Autodesk Inventor part; units mm, degrees
ref_plane "YZ Plane" through (0, 0, 0) normal (1, 0, 0) x (0, 1, 0)
ref_plane "XZ Plane" through (0, 0, 0) normal (0, 1, 0) x (-1, 0, 0)
ref_plane "XY Plane" through (0, 0, 0) normal (0, 0, 1) x (1, 0, 0)
sketch "Sketch1" plane through (0, 0, 0) normal (0, 1, 0) x (-1, 0, 0)
  line L0 (20, 147) -> (20, 150)
  line L1 (20, 150) -> (40, 150)
  line L2 (40, 150) -> (40, 147)
  line L3 (-20, 147) -> (-20, 150)
  line L4 (-20, 150) -> (-40, 150)
  line L5 (-40, 150) -> (-40, 147)
  line L6 (-40, 147) -> (-57, 147)
  line L7 (57, 147) -> (40, 147)
  line L8 (20, 147) -> (-20, 147)
  line L9 (20, -147) -> (20, -150)
  line L10 (20, -150) -> (40, -150)
  line L11 (40, -150) -> (40, -147)
  line L12 (-40, -147) -> (-40, -150)
  line L13 (-40, -150) -> (-20, -150)
  line L14 (-20, -150) -> (-20, -147)
  line L15 (40, -147) -> (57, -147)
  line L16 (-57, -147) -> (-40, -147)
  line L17 (-20, -147) -> (20, -147)
  line L18 (-57, 131.4286) -> (-60, 131.4286)
  line L19 (-60, 131.4286) -> (-60, 108.5714)
  line L20 (-60, 108.5714) -> (-57, 108.5714)
  line L21 (-57, 11.4286) -> (-60, 11.4286)
  line L22 (-60, 11.4286) -> (-60, -11.4286)
  line L23 (-60, -11.4286) -> (-57, -11.4286)
  line L24 (-57, -108.5714) -> (-60, -108.5714)
  line L25 (-60, -108.5714) -> (-60, -131.4286)
  line L26 (-60, -131.4286) -> (-57, -131.4286)
  line L27 (-57, 147) -> (-57, 131.4286)
  line L28 (-57, -131.4286) -> (-57, -147)
  line L29 (57, 131.4286) -> (60, 131.4286)
  line L30 (60, 131.4286) -> (60, 108.5714)
  line L31 (60, 108.5714) -> (57, 108.5714)
  line L32 (57, 11.4286) -> (60, 11.4286)
  line L33 (60, 11.4286) -> (60, -11.4286)
  line L34 (60, -11.4286) -> (57, -11.4286)
  line L35 (57, -108.5714) -> (60, -108.5714)
  line L36 (60, -108.5714) -> (60, -131.4286)
  line L37 (60, -131.4286) -> (57, -131.4286)
  line L38 (57, 131.4286) -> (57, 147)
  line L39 (57, 11.4286) -> (57, 108.5714)
  line L40 (57, -147) -> (57, -131.4286)
  line L41 (57, -108.5714) -> (57, -11.4286)
  line L42 (-57, 57.1429) -> (-60, 57.1429)
  line L43 (-60, 57.1429) -> (-60, 34.2857)
  line L44 (-60, 34.2857) -> (-57, 34.2857)
  line L45 (-57, -34.2857) -> (-60, -34.2857)
  line L46 (-60, -34.2857) -> (-60, -57.1429)
  line L47 (-60, -57.1429) -> (-57, -57.1429)
  line L48 (-57, 108.5714) -> (-57, 57.1429)
  line L49 (-57, 34.2857) -> (-57, 11.4286)
  line L50 (-57, -11.4286) -> (-57, -34.2857)
  line L51 (-57, -57.1429) -> (-57, -108.5714)
  line L52 (-36, 80) -> (-12, 80)
  line L53 (-12, 80) -> (-12, 83)
  line L54 (-12, 83) -> (-36, 83)
  line L55 (-36, 83) -> (-36, 80)
  line L56 (-36, -80) -> (-12, -80)
  line L57 (-12, -80) -> (-12, -83)
  line L58 (-12, -83) -> (-36, -83)
  line L59 (-36, -83) -> (-36, -80)
  line L60 (12, 83) -> (36, 83)
  line L61 (36, 83) -> (36, 80)
  line L62 (36, 80) -> (12, 80)
  line L63 (12, 80) -> (12, 83)
  line L64 (12, -80) -> (36, -80)
  line L65 (36, -80) -> (36, -83)
  line L66 (36, -83) -> (12, -83)
  line L67 (12, -83) -> (12, -80)
  point P0 (0, 0)
  point P1 (-60, 120)
  point P2 (-60, -120)
  dimension "d1" = 294
  dimension "d5" = 20
  dimension "d7" = 20
  dimension "d9" = 3
  dimension "d10" = 147
  dimension "d11" = 3
  dimension "d12" = 57
  dimension "d13" = 3
  dimension "d14" = 17
  dimension "d15" = 3
  dimension "d16" = 17
  dimension "d17" = 22.8571
  dimension "d18" = 11.4286
  dimension "d20" = 120
  dimension "d21" = 17
  dimension "d24" = 114
  dimension "d25" = 22.8571
  dimension "d26" = 24
  dimension "d27" = 3
  dimension "d28" = 3
  dimension "d29" = 22.8571
  dimension "d30" = 24
  dimension "d31" = 24
  dimension "d32" = 22.8571
  dimension "d33" = 120
extrude "Extrusion1" add sketch "Sketch1" along normal blind 3
sketch "Sketch2" plane through (0, 3, 0) normal (0, 1, 0) x (1, 0, 0)
  line L0 (34.2, 76.5) -> (11.4, 76.5)
  line L1 (11.4, 76.5) -> (11.4, 73.5)
  line L2 (11.4, 73.5) -> (34.2, 73.5)
  line L3 (34.2, 73.5) -> (34.2, 76.5)
  line L4 (-11.4, 76.5) -> (-34.2, 76.5)
  line L5 (-34.2, 76.5) -> (-34.2, 73.5)
  line L6 (-34.2, 73.5) -> (-11.4, 73.5)
  line L7 (-11.4, 73.5) -> (-11.4, 76.5)
  line L8 (34.2, 73.5) -> (57, 73.5) construction
  line L9 (11.4, 73.5) -> (-11.4, 73.5) construction
  line L10 (-34.2, 73.5) -> (-57, 73.5) construction
  line L11 (-57, 108.5714) -> (-57, 11.4286)
  line L12 (57, 57.1429) -> (57, 108.5714)
  point P0 (0, 0)
  dimension "d34" = 22.8
  dimension "d35" = 22.8
  dimension "d36" = 3
  dimension "d37" = 73.5
extrude "Extrusion2" cut sketch "Sketch2" against normal through all
pattern_linear "Rectangular Pattern1" count 3 spacing 75 along (0, 0, 1) of "Extrusion2"
equation "\"d1\" = wt - 2 * tt"
equation "\"d9\" = tt"
equation "\"d11\" = tt"
equation "\"d13\" = tt"
equation "\"d15\" = tt"
equation "\"d17\" = 0.142857 * shelfW + 2 * tol"
equation "\"d24\" = ht - 2 * tt"
equation "\"d25\" = 0.142857 * shelfW - 2 * tol"
equation "\"d26\" = 0.2 * ht + 2 * tol"
equation "\"d27\" = tt"
equation "\"d28\" = tt"
equation "\"d29\" = 0.142857 * shelfW - tol"
equation "\"d30\" = 0.2 * ht - tol"
equation "\"d31\" = 0.2 * ht - 2 * tol"
equation "\"d32\" = 0.142857 * shelfW - tol"
equation "\"d22\" = tt"
equation "\"d34\" = -0.4 * tt + 0.2 * ht + 2 * tol"
equation "\"d36\" = tt"
equation "\"d42\" = 0.25 * wt"
equation "\"d0\" = 0.5 * wt - tt"
equation "\"tt\" = 3"
equation "\"tol\" = 0"
equation "\"tiroir\" = 1"
equation "\"nHoles\" = 4"
equation "\"shelfH\" = 35"
equation "\"d3\" = 0.5 * ht - tt"
properties part number "in_separator"
Geometry: final body of the model. Coordinates: model frame, mm. Give positions to 0.01 mm unless a question says otherwise; leave off trailing zeros. Order: outer loops, then holes, each group sorted by start corner. A loop starts at its lowest first (then second) coordinate and runs counter-clockwise, first axis right, second up. Notation, with made-up numbers: (0, -4.5) -> (28, -4.5) arc R32 cw to (28, 22.5) -> close; hole circle Ø1 at (20.25, -38.75). An arc over 180 degrees is marked (long way). Write each question's results on one line, items separated by ' | '.
1) Line query: line 1 along Z through (x, y) = (18, 2.3); line 2 along X through (y, z) = (2.15, 49.5); line 3 along Z through (x, y) = (-53, 0.2). Output: solid intervals per line, ascending.
Geometry says:
line 1: z = -147 to -83, -80 to -76.5, -73.5 to -1.5, 1.5 to 73.5, 76.5 to 80, 83 to 147 | line 2: x = -57 to 60 | line 3: z = -147 to 147
2) Cut plane A-A (x = 25.5). Output: boundary loops of the cut face in (y, z), and give its area (3 significant figures).
Geometry says:
outline: (0, -150) -> (3, -150) -> (3, -83) -> (0, -83) -> close; (0, -80) -> (3, -80) -> (3, -76.5) -> (0, -76.5) -> close; (0, -73.5) -> (3, -73.5) -> (3, -1.5) -> (0, -1.5) -> close; (0, 1.5) -> (3, 1.5) -> (3, 73.5) -> (0, 73.5) -> close; (0, 76.5) -> (3, 76.5) -> (3, 80) -> (0, 80) -> close; (0, 83) -> (3, 83) -> (3, 150) -> (0, 150) -> close | area: 855 mm²
3) Cut plane B-B (z = -105). Output: boundary loops of the cut face in (x, y).
Geometry says:
outline: (-57, 0) -> (57, 0) -> (57, 3) -> (-57, 3) -> close
4) First-contact query: pin 1 Ø1.5 at (x, y) = (1.5, 1.5) entering from -Z; pin 2 Ø1 at (y, z) = (2, 66.5) entering from -X; pin 3 Ø1.5 at (x, y) = (-58, 2) entering from -Z. Flat tips, straight axial feed; report the tip coordinate or a pass-through.
Geometry says:
pin 1: stops at z = -147 | pin 2: stops at x = -57 | pin 3: stops at z = -131.43
5) Cut plane D-D (x = 4). Output: boundary loops of the cut face in (y, z), and give its area (3 significant figures).
Geometry says:
outline: (0, -147) -> (3, -147) -> (3, 147) -> (0, 147) -> close | area: 882 mm²
6) Cut plane C-C (y = 1.7). Give the number of separate pieces and of enclosed holes in the cut face, and give its area (3 significant figures).
Geometry says:
separate pieces: 1 | enclosed holes: 10 | area: 33,600 mm²
